Can you work these out from the drawing? Everything is in mm from the part's minimum corner. A direction names the side the tool comes from. Round coordinates to 2 decimals unless told otherwise and drop trailing zeros. Write each loop counter-clockwise with the first axis right and the second up, starting at its lowest first coordinate (ties: lowest second). Pieces come first, ordered by that corner, then holes.
Q1. If we section it at C-C (y = 83.5): Please give me the cut outline in (x, z).
Q2. For the marked faces 1 and 2, which set-ups out of +Z, -Z, +X, -X, +Y, -Y let a thin tool reach every point of the face, with its end or its side?
Q3. I'm going to push flat-ended pins straight in: pin 1 Ø12 at (x, z) = (136, 110.5) entering from -Y; pin 2 Ø2.5 at (x, y) = (231, 54.5) entering from -Z; pin 3 Ø4 at (x, z) = (228.5, 79.5) entering from -Y. Where does each tip first touch, or does it pass through?
Q4. If we section it at A-A (z = 59): Please give me the cut outline in (x, y), plus the area to 3 significant figures.
Q5. Please list where these lines run through material, in increasing order: line 1 along X through (y, z) = (119.5, 82); line 2 along Y through (x, z) = (156, 41.5).
Q6. If we section it at B-B (x = 65): Please give me the cut outline in (y, z).
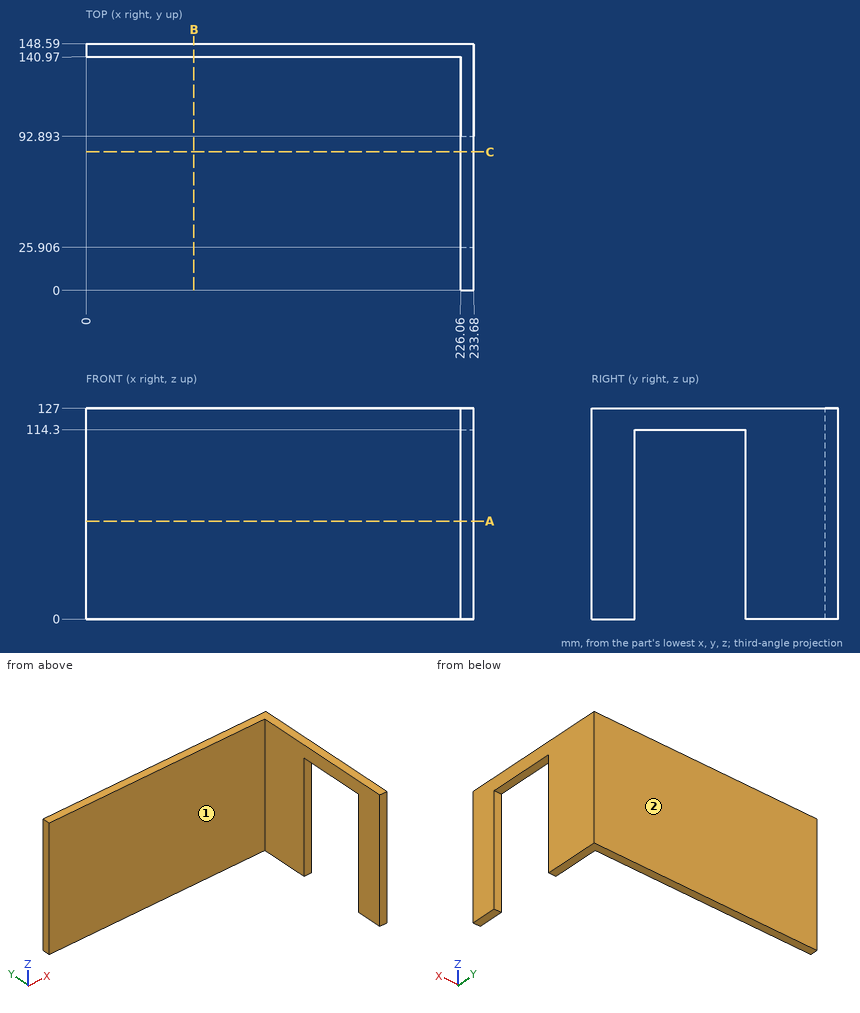
A:
1. outline: (226.06, 114.3) - (233.68, 114.3) - (233.68, 127) - (226.06, 127) - close
2. face 1: +Z, -Z, -X, -Y
2. face 2: +Z, -Z, +X, -X, +Y
3. pin 1: stops at y = 140.97
3. pin 2: stops at z = 114.3
3. pin 3: stops at y = 0
4. outline: (0, 140.97) - (226.06, 140.97) - (226.06, 92.89) - (233.68, 92.89) - (233.68, 148.59) - (0, 148.59) - close; (226.06, 0) - (233.68, 0) - (233.68, 25.91) - (226.06, 25.91) - close
4. area: 2,340 mm2
5. line 1: x = 226.06 to 233.68
5. line 2: y = 140.97 to 148.59
6. outline: (140.97, 0) - (148.59, 0) - (148.59, 127) - (140.97, 127) - close
